```python
from build123d import *

# Parameters (mm, degrees)
BOSS_EXTRUDE1_START = 0.5
SKETCH1_W           = 25
SKETCH1_H           = 14
BOSS_EXTRUDE1_DEPTH = 2
SKETCH2_W           = 25
SKETCH2_H           = 2.1
BOSS_EXTRUDE2_DEPTH = 6
SKETCH3_W           = 40
SKETCH3_H           = 42
BOSS_EXTRUDE3_DEPTH = 4
BOSS_EXTRUDE5_START = -18.3
SKETCH4_2_R         = 1.5
BOSS_EXTRUDE5_DEPTH = 4
SKETCH5_W           = 40
SKETCH5_H           = 18.3
BOSS_EXTRUDE6_DEPTH = 5.3
SKETCH7_R           = 4.5
CUT_EXTRUDE1_DEPTH  = 4
SKETCH9_W           = 35.343646405
SKETCH9_H           = 8.813303651
CUT_EXTRUDE3_DEPTH  = 10
SKETCH11_R          = 12.5
SKETCH11_R_2        = 1.5
SKETCH11_R_3        = 3.55
BOSS_EXTRUDE7_DEPTH = 4
SKETCH12_R          = 12.5
BOSS_EXTRUDE8_DEPTH = 14
SKETCH13_W          = 15
SKETCH13_H          = 2.1
BOSS_EXTRUDE9_DEPTH = 6
CUT_EXTRUDE2_DEPTH  = 64.84830294
SKETCH14_W          = 6.01632357
SKETCH14_H          = 22.957747356
CUT_EXTRUDE4_DEPTH  = 64.347816028


# Read off the part's stored shape, not the designer's step: CSK for M4 Flat Head Machine Screw1
with BuildPart() as part:
    # Sketch1 → Boss-Extrude1 (new body)
    with BuildSketch(Plane.XY.offset(-1).offset(BOSS_EXTRUDE1_START)):
        with Locations((23.192657344, 4)):
            Rectangle(SKETCH1_W, SKETCH1_H)
    extrude(amount=BOSS_EXTRUDE1_DEPTH)

    # Sketch2 → Boss-Extrude2 (add)
    with BuildSketch(Plane(origin=(0, 0, -0.5), x_dir=(-1, 0, 0), z_dir=(0, 0, -1))):
        with Locations((-23.192657344, 9.95)):
            Rectangle(SKETCH2_W, SKETCH2_H)
        with Locations((-23.192657344, -1.95)):
            Rectangle(SKETCH2_W, SKETCH2_H)
    extrude(amount=BOSS_EXTRUDE2_DEPTH)

    # Sketch3 → Boss-Extrude3 (add)
    with BuildSketch(Plane(origin=(0, 0, -0.5), x_dir=(-1, 0, 0), z_dir=(0, 0, -1))):
        with Locations((-15.692657344, 18)):
            Rectangle(SKETCH3_W, SKETCH3_H)
    extrude(amount=-BOSS_EXTRUDE3_DEPTH)

    # Sketch4<2> → Boss-Extrude5 (add)
    with BuildSketch(Plane(origin=(0, 35, 0), x_dir=(1, 0, 0), z_dir=(0, 1, 0)).offset(BOSS_EXTRUDE5_START)):
        with BuildLine():
            Line((-1.349302764, 24.5), (-1.349302764, 0.5))
            Line((-1.349302764, 0.5), (8.650697236, 0.5))
            Line((8.650697236, 0.5), (8.650697236, 24.5))
            ThreePointArc((8.650697236, 24.5), (3.650697236, 29.5), (-1.349302764, 24.5))
        make_face()
        with Locations(Location((3.650697236, 7.5, 0), (0, 0, 270))):
            Circle(SKETCH4_2_R, mode=Mode.SUBTRACT)
        with Locations(Location((3.650697236, 24.5, 0), (0, 0, 270))):
            Circle(SKETCH4_2_R, mode=Mode.SUBTRACT)
    extrude(amount=-BOSS_EXTRUDE5_DEPTH)

    # Sketch5 → Boss-Extrude6 (add)
    with BuildSketch(Plane(origin=(0, 0, -0.5), x_dir=(-1, 0, 0), z_dir=(0, 0, -1))):
        with Locations((-15.692657344, 25.85)):
            Rectangle(SKETCH5_W, SKETCH5_H)
    extrude(amount=BOSS_EXTRUDE6_DEPTH)

    # CSK for M4 Flat Head Machine Screw1 outl → CSK for M4 Flat Head Machine Screw1 (revolve, cut)
    with BuildSketch(Plane(origin=(15.942657344, 23.75, 0), x_dir=(1, 0, 0), z_dir=(0, -1, 0))):
        Polygon((2.25, -3.35), (2.25, 3.5), (0, 3.5), (0, -5.8), (4.7, -5.8), align=None)
    revolve(axis=Axis((15.942657344, 23.75, 0), (0, 0, 1)), mode=Mode.SUBTRACT)

    # CSK for M4 Flat Head Machine Screw1 2 ou → CSK for M4 Flat Head Machine Screw1 2 (revolve, cut)
    with BuildSketch(Plane(origin=(15.942657344, 3.75, 0), x_dir=(1, 0, 0), z_dir=(0, -1, 0))):
        Polygon((4.7, -0.5), (2.25, 1.95), (2.25, 3.5), (0, 3.5), (0, -0.5), align=None)
    revolve(axis=Axis((15.942657344, 3.75, 0), (0, 0, 1)), mode=Mode.SUBTRACT)

    # CSK for M4 Flat Head Machine Screw1 3 ou → CSK for M4 Flat Head Machine Screw1 3 (revolve, cut)
    with BuildSketch(Plane(origin=(15.942657344, 13.75, 0), x_dir=(1, 0, 0), z_dir=(0, -1, 0))):
        Polygon((4.7, -0.5), (2.25, 1.95), (2.25, 3.5), (0, 3.5), (0, -0.5), align=None)
    revolve(axis=Axis((15.942657344, 13.75, 0), (0, 0, 1)), mode=Mode.SUBTRACT)

    # CSK for M4 Flat Head Machine Screw1 4 ou → CSK for M4 Flat Head Machine Screw1 4 (revolve, cut)
    with BuildSketch(Plane(origin=(25.942657344, 13.75, 0), x_dir=(1, 0, 0), z_dir=(0, -1, 0))):
        Polygon((2.25, 1.95), (2.25, 3.5), (0, 3.5), (0, -0.5), (4.7, -0.5), align=None)
    revolve(axis=Axis((25.942657344, 13.75, 0), (0, 0, 1)), mode=Mode.SUBTRACT)

    # Sketch7 → Cut-Extrude1 (cut)
    with BuildSketch(Plane(origin=(0, 0, 3.5), x_dir=(-1, 0, 0), z_dir=(0, 0, -1))):
        with Locations((-35.792657344, 33.75)):
            Circle(SKETCH7_R)
        with Locations((3.907342656, 33.75)):
            Circle(SKETCH7_R)
        with Locations((3.907342656, -6.25)):
            Circle(SKETCH7_R)
        with Locations((-35.792657344, -6.25)):
            Circle(SKETCH7_R)
    extrude(amount=CUT_EXTRUDE1_DEPTH, mode=Mode.SUBTRACT)

    # Sketch9 → Cut-Extrude3 (cut)
    with BuildSketch(Plane.ZY.offset(1.349302764)):
        with Locations((-18.171823203, 12.293348175)):
            Rectangle(SKETCH9_W, SKETCH9_H)
    extrude(amount=-CUT_EXTRUDE3_DEPTH, mode=Mode.SUBTRACT)

    # Sketch11 → Boss-Extrude7 (add)
    # profile 1 of 4: a face of its own
    with BuildSketch(Plane.XZ.offset(-16.7)):
        with BuildLine():
            Line((6.787532506, -5.8), (-4.307342656, -5.8))
            Line((-4.307342656, -5.8), (-4.807342656, -5.8))
            Line((-4.807342656, -5.8), (-4.807342656, -20.8))
            ThreePointArc((-4.807342656, -20.8), (-1.570691199, -11.320533638), (6.787532506, -5.8))
        make_face()
    # profile 2 of 4: a face of its own
    with BuildSketch(Plane.XZ.offset(-16.7)):
        with BuildLine():
            Line((14.597782182, -5.8), (6.787532506, -5.8))
            ThreePointArc((6.787532506, -5.8), (-1.570691199, -11.320533638), (-4.807342656, -20.8))
            ThreePointArc((-4.807342656, -20.8), (10.692657344, -36.3), (26.192657344, -20.8))
            ThreePointArc((26.192657344, -20.8), (22.956005887, -11.320533638), (14.597782182, -5.8))
        make_face()
        with Locations((10.692657344, -20.8)):
            Circle(SKETCH11_R, mode=Mode.SUBTRACT)
    # profile 3 of 4: a face of its own
    with BuildSketch(Plane.XZ.offset(-16.7)):
        with Locations((10.692657344, -20.8)):
            Circle(SKETCH11_R)
        with Locations(Location((10.692657344, -12.3, 0), (0, 0, 270))):
            Circle(SKETCH11_R_2, mode=Mode.SUBTRACT)
        with Locations(Location((10.692657344, -20.8, 0), (0, 0, 270))):
            Circle(SKETCH11_R_3, mode=Mode.SUBTRACT)
        with Locations(Location((19.192657344, -20.8, 0), (0, 0, 270))):
            Circle(SKETCH11_R_2, mode=Mode.SUBTRACT)
        with Locations(Location((10.692657344, -29.3, 0), (0, 0, 270))):
            Circle(SKETCH11_R_2, mode=Mode.SUBTRACT)
        with Locations(Location((2.192657344, -20.8, 0), (0, 0, 270))):
            Circle(SKETCH11_R_2, mode=Mode.SUBTRACT)
    # profile 4 of 4: a face of its own
    with BuildSketch(Plane.XZ.offset(-16.7)):
        with BuildLine():
            Line((26.192657344, -5.8), (14.597782182, -5.8))
            ThreePointArc((14.597782182, -5.8), (22.956005887, -11.320533638), (26.192657344, -20.8))
            Line((26.192657344, -20.8), (26.192657344, -5.8))
        make_face()
    extrude(amount=-BOSS_EXTRUDE7_DEPTH)

    # Sketch12 → Boss-Extrude8 (add)
    # profile 1 of 3: a face of its own
    with BuildSketch(Plane(origin=(0, 20.7, 0), x_dir=(1, 0, 0), z_dir=(0, 1, 0))):
        with BuildLine():
            ThreePointArc((26.192657344, 20.8), (10.692657344, 36.3), (-4.807342656, 20.8))
            ThreePointArc((-4.807342656, 20.8), (-1.570691199, 11.320533638), (6.787532506, 5.8))
            Line((6.787532506, 5.8), (12.366695935, 5.8))
            Line((12.366695935, 5.8), (14.597782182, 5.8))
            ThreePointArc((14.597782182, 5.8), (22.956005887, 11.320533638), (26.192657344, 20.8))
        make_face()
        with Locations(Location((10.692657344, 20.8, 0), (0, 0, 270))):
            Circle(SKETCH12_R, mode=Mode.SUBTRACT)
    # profile 2 of 3: a face of its own
    with BuildSketch(Plane(origin=(0, 20.7, 0), x_dir=(1, 0, 0), z_dir=(0, 1, 0))):
        with BuildLine():
            Line((-4.807342656, 20.8), (-4.807342656, 5.8))
            Line((-4.807342656, 5.8), (-4.307342656, 5.8))
            Line((-4.307342656, 5.8), (6.787532506, 5.8))
            ThreePointArc((6.787532506, 5.8), (-1.570691199, 11.320533638), (-4.807342656, 20.8))
        make_face()
    # profile 3 of 3: a face of its own
    with BuildSketch(Plane(origin=(0, 20.7, 0), x_dir=(1, 0, 0), z_dir=(0, 1, 0))):
        with BuildLine():
            Line((26.192657344, 5.8), (26.192657344, 20.8))
            ThreePointArc((26.192657344, 20.8), (22.956005887, 11.320533638), (14.597782182, 5.8))
            Line((14.597782182, 5.8), (19.518618753, 5.8))
            Line((19.518618753, 5.8), (26.192657344, 5.8))
        make_face()
    extrude(amount=BOSS_EXTRUDE8_DEPTH)

    # Sketch13 → Boss-Extrude9 (add)
    with BuildSketch(Plane(origin=(0, 0, -0.5), x_dir=(-1, 0, 0), z_dir=(0, 0, -1))):
        with Locations((-3.192657344, 9.95)):
            Rectangle(SKETCH13_W, SKETCH13_H)
        with Locations((-3.192657344, -1.95)):
            Rectangle(SKETCH13_W, SKETCH13_H)
    extrude(amount=BOSS_EXTRUDE9_DEPTH)

    # Sketch8 → Cut-Extrude2 (cut, through all)
    with BuildSketch(Plane(origin=(0, 0, -0.5), x_dir=(-1, 0, 0), z_dir=(0, 0, -1))):
        with BuildLine():
            ThreePointArc((-12.283764069, 16.7), (-15.942657344, 18.45), (-19.601550619, 16.7))
            ThreePointArc((-19.601550619, 16.7), (-20.640973864, 13.875785056), (-19.754153113, 11))
            ThreePointArc((-19.754153113, 11), (-15.942657344, 9.05), (-12.131161575, 11))
            ThreePointArc((-12.131161575, 11), (-11.244340824, 13.875785056), (-12.283764069, 16.7))
        make_face()
        with BuildLine():
            ThreePointArc((-22.283764069, 16.7), (-25.942657344, 18.45), (-29.601550619, 16.7))
            ThreePointArc((-29.601550619, 16.7), (-30.640973864, 13.875785056), (-29.754153113, 11))
            ThreePointArc((-29.754153113, 11), (-25.942657344, 9.05), (-22.131161575, 11))
            ThreePointArc((-22.131161575, 11), (-21.244340824, 13.875785056), (-22.283764069, 16.7))
        make_face()
    extrude(amount=CUT_EXTRUDE2_DEPTH, mode=Mode.SUBTRACT)

    # Sketch14 → Cut-Extrude4 (cut, through all)
    with BuildSketch(Plane(origin=(0, 34.7, 0), x_dir=(1, 0, 0), z_dir=(0, 1, 0))):
        with Locations((-7.315504441, 17.278873678)):
            Rectangle(SKETCH14_W, SKETCH14_H)
    extrude(amount=-CUT_EXTRUDE4_DEPTH, mode=Mode.SUBTRACT)


solid = part.part
```
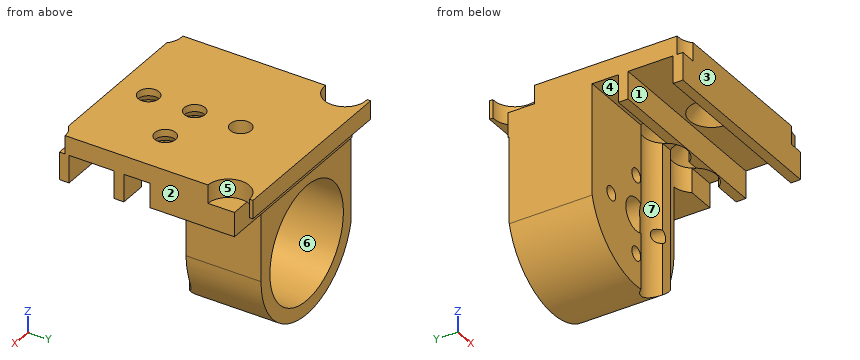
Build history of the part. All positions in model axes, mm. Face numbers are marked on the shaded views. A direction names the side the tool comes from. Round coordinates to 2 decimals unless told otherwise and drop trailing zeros. Write each loop counter-clockwise with the first axis right and the second up, starting at its lowest first coordinate (ties: lowest second). Pieces come first, ordered by that corner, then holes. Notation, with made-up numbers: (49, -4) - (96, -4) arc R18 cw to (96, 19) - close; hole circle Ø10 at (86, 86.25). An arc over 180 degrees is marked (long way). Write each question's results on one line, items separated by ' | '. Start each with the question number.
Item 1: Saw through at B-B (y = 13.75). Write the cut outline in (x, z), and give its area (3 significant figures).
Item 2: Saw through at C-C (z = -12.3). Write the cut outline in (x, y).
Item 3: Saw through at D-D (y = 23.75). Write the cut outline in (x, z), and give its area (3 significant figures).
Item 4: Drop flat-ended pins along their axis: P1, Ø4, axis at x = 15.94, y = 13.75, coming from the -Z side; P2, Ø4, axis at x = 10.69, z = -29.3, coming from the -Y side; P3, Ø6, axis at x = 24.5, y = 28, coming from the -Z side; P4, Ø8, axis at y = 33.5, z = -32, coming from the -X side. Give the stop position or say it passes through.
Item 5: Wall check: L1, parallel to Y at x = 7, z = -1.5; L2, parallel to Z at x = 33.5, y = 21; L3, parallel to Z at x = 20, y = 10.5. Give the ranges that are in metal, low to high. Write a range as [from, to].
Item 6: Which spindle directions (+Z, -Z, +X, -X, +Y, -Y) get a long thin tool onto all of the face, cutting with end or side? Do the marked faces 4, 5, 6 and 7. Say none if no direction does.
Item 7: Mould opens along Y. For the marked faces 1, 2 and 3 say: pulls with the +Y half, pulls with the -Y half, needs draft (parallel to the pull), parting line crosses it, or undercut.
Item 8: Saw through at A-A (y = 3.75). Write the cut outline in (x, z).
Results are:
1) outline: (-4.31, -0.5) - (11.24, -0.5) - (13.69, 1.95) - (13.69, 3.5) - (-4.31, 3.5) - close; (18.19, 1.95) - (20.64, -0.5) - (21.24, -0.5) - (23.69, 1.95) - (23.69, 3.5) - (18.19, 3.5) - close; (28.19, 1.95) - (30.64, -0.5) - (35.69, -0.5) - (35.69, 3.5) - (28.19, 3.5) - close | area: 112 mm²
2) outline: (-4.31, 16.7) - (9.19, 16.7) - (9.19, 20.7) - (1.53, 20.7) - (1.53, 34.7) - (-4.31, 34.7) - close; (12.19, 16.7) - (12.28, 16.7) arc R4.7 cw to (19.6, 16.7) - (22.28, 16.7) arc R4.7 cw to (26.19, 18.44) - (26.19, 34.7) - (19.86, 34.7) - (19.86, 20.7) - (12.19, 20.7) - close
3) outline: (-4.31, -24.71) arc R15.5 ccw to (26.19, -20.8) - (26.19, -5.8) - (35.69, -5.8) - (35.69, 3.5) - (18.19, 3.5) - (18.19, -3.35) - (20.64, -5.8) - (11.24, -5.8) - (13.69, -3.35) - (13.69, 3.5) - (-4.31, 3.5) - close; hole circle Ø25 at (10.69, -20.8) | area: 667 mm²
4) P1: passes through | P2: stops at y = 16.7 | P3: stops at z = -31.91 | P4: stops at x = -3.03
5) L1: y = [-3, -0.9], [8.9, 11], [16.7, 35] | L2: z = [-5.8, 3.5] | L3: z = [-6.5, 3.5]
6) face 4: -Z, +X, -X | face 5: +Z, +X | face 6: +Y | face 7: -Z
7) face 1: undercut | face 2: needs draft | face 3: pulls with the -Y half
8) outline: (-4.31, -0.5) - (11.24, -0.5) - (13.69, 1.95) - (13.69, 3.5) - (-4.31, 3.5) - close; (18.19, 1.95) - (20.64, -0.5) - (35.69, -0.5) - (35.69, 3.5) - (18.19, 3.5) - close
